Drawing for the job (mm, zero at the part's lowest x, y, z). Give positions to 0.01 mm unless a question says otherwise; leave off trailing zeros. Order: outer loops, then holes, each group sorted by start corner. A loop starts at its lowest first (then second) coordinate and runs counter-clockwise, first axis right, second up. Notation, with made-up numbers: (36.25, 19) -> (57.25, 19) arc R24 ccw to (57.25, 55) -> close; hole circle Ø2 at (20, 33.5). An arc over 180 degrees is marked (long way). Use one line per item in the form item = value. Start each with the question number.
1) Cut at A-A, the plane x = 7.5. Give the cut face in (y, z), and give its area (4 significant figures).
2) Cut at B-B, the plane z = 7.5. Give the cut face in (x, y), and give its area (4 significant figures).
3) Probe line 1 (Y direction, x = 9, z = 12.75); line 2 (Z direction, x = 7, y = 63.5); line 3 (X direction, y = 100, z = 9.5). List the from-to ranges inside material, lowest first.
4) Cut at C-C, the plane y = 68.5. Give the cut face in (x, z), and give its area (3 significant figures).
5) Drop flat-ended pins along their axis: P1, Ø1.5, axis at x = 12.5, y = 126, coming from the -Z side; P2, Ø2, axis at y = 62, z = 8, coming from the +X side; P3, Ø2, axis at y = 63, z = 12, coming from the -X side. Give the stop position or say it passes through.
6) Mould opens along Y. For the marked faces 1, 2, 3 and 4 say: pulls with the +Y half, pulls with the -Y half, needs draft (parallel to the pull), parting line crosses it, or undercut.
7) Cut at D-D, the plane y = 11. Give the cut face in (x, z).
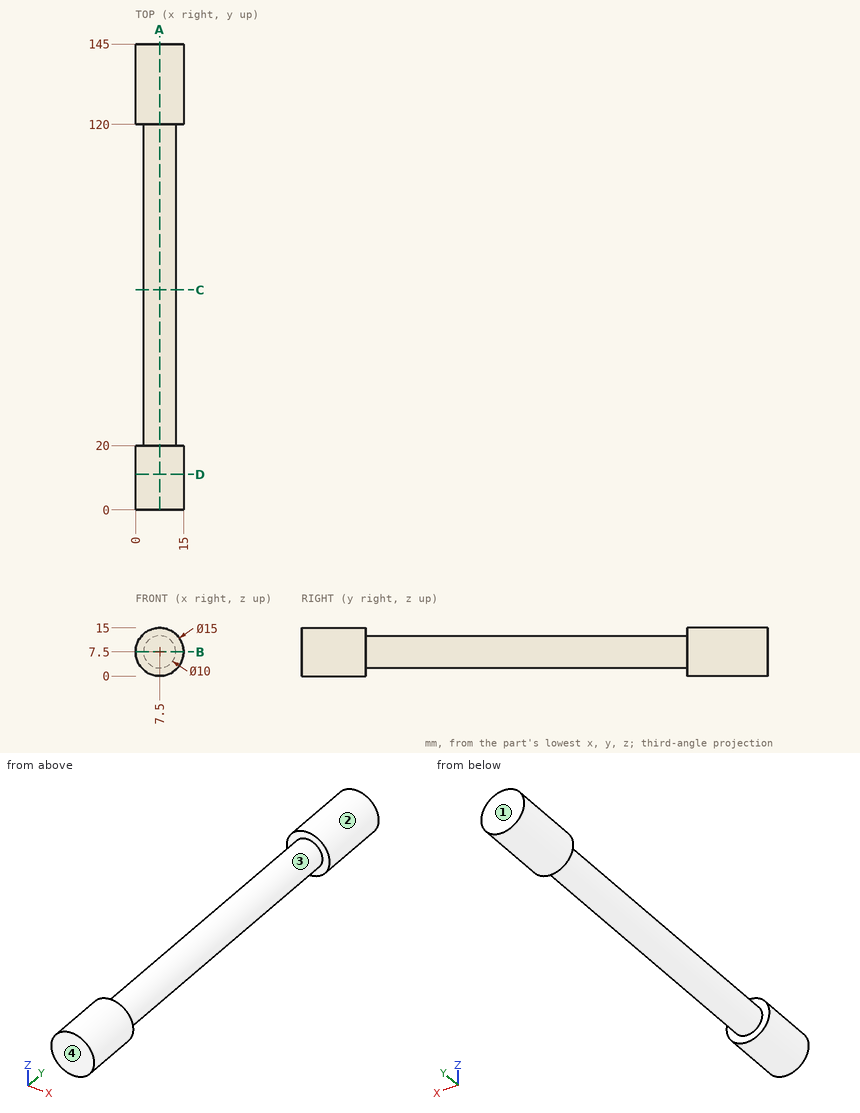
Result:
q1.outline = (0, 0) -> (20, 0) -> (20, 2.5) -> (120, 2.5) -> (120, 0) -> (145, 0) -> (145, 15) -> (120, 15) -> (120, 12.5) -> (20, 12.5) -> (20, 15) -> (0, 15) -> close
q1.area = 1,675 mm²
q2.outline = (0, 0) -> (15, 0) -> (15, 20) -> (12.5, 20) -> (12.5, 120) -> (15, 120) -> (15, 145) -> (0, 145) -> (0, 120) -> (2.5, 120) -> (2.5, 20) -> (0, 20) -> close
q2.area = 1,675 mm²
q3.line_1 = 0 to 20, 120 to 145
q3.line_2 = 2.53 to 12.47
q3.line_3 = 2.92 to 12.08
q4.outline = circle Ø10 at (7.5, 7.5)
q4.area = 78.5 mm²
q5.P1 = 1.32
q5.P2 = 12.5
q5.P3 = 3.93
q6.face_1 = pulls with the +Y half
q6.face_2 = needs draft
q6.face_3 = undercut
q6.face_4 = pulls with the -Y half
q7.outline = circle Ø15 at (7.5, 7.5)
